```python
from build123d import *

# Parameters (mm, degrees)
SKETCH1_W           = 100
SKETCH1_H           = 75
BOSS_EXTRUDE1_DEPTH = 1.5875
SKETCH4_R           = 1.35
CUT_EXTRUDE1_DEPTH  = 2.5875


with BuildPart() as part:
    # Sketch1 → Boss-Extrude1 (new body)
    with BuildSketch(Plane(origin=(0, 0, 0), x_dir=(1, 0, 0), z_dir=(0, 1, 0))):
        with Locations((50, 37.5)):
            Rectangle(SKETCH1_W, SKETCH1_H)
    extrude(amount=BOSS_EXTRUDE1_DEPTH)

    # Sketch4 → Cut-Extrude1 (cut, through all)
    with BuildSketch(Plane(origin=(0, 1.5875, 0), x_dir=(1, 0, 0), z_dir=(0, 1, 0))):
        with Locations((10.86, 53.96)):
            Circle(SKETCH4_R)
        with Locations((10.86, 49.96)):
            Circle(SKETCH4_R)
        with Locations((10.86, 45.96)):
            Circle(SKETCH4_R)
        with Locations((14.86, 53.96)):
            Circle(SKETCH4_R)
        with Locations((14.86, 49.96)):
            Circle(SKETCH4_R)
        with Locations((14.86, 45.96)):
            Circle(SKETCH4_R)
        with Locations((18.86, 53.96)):
            Circle(SKETCH4_R)
        with Locations((18.86, 49.96)):
            Circle(SKETCH4_R)
        with Locations((18.86, 45.96)):
            Circle(SKETCH4_R)
        with Locations((34.86, 53.96)):
            Circle(SKETCH4_R)
        with Locations((34.86, 49.96)):
            Circle(SKETCH4_R)
        with Locations((34.86, 45.96)):
            Circle(SKETCH4_R)
        with Locations((38.86, 53.96)):
            Circle(SKETCH4_R)
        with Locations((38.86, 49.96)):
            Circle(SKETCH4_R)
        with Locations((38.86, 45.96)):
            Circle(SKETCH4_R)
        with Locations((42.86, 53.96)):
            Circle(SKETCH4_R)
        with Locations((42.86, 49.96)):
            Circle(SKETCH4_R)
        with Locations((42.86, 45.96)):
            Circle(SKETCH4_R)
        with Locations((58.86, 53.96)):
            Circle(SKETCH4_R)
        with Locations((58.86, 49.96)):
            Circle(SKETCH4_R)
        with Locations((58.86, 45.96)):
            Circle(SKETCH4_R)
        with Locations((62.86, 53.96)):
            Circle(SKETCH4_R)
        with Locations((62.86, 49.96)):
            Circle(SKETCH4_R)
        with Locations((62.86, 45.96)):
            Circle(SKETCH4_R)
        with Locations((66.86, 53.96)):
            Circle(SKETCH4_R)
        with Locations((66.86, 49.96)):
            Circle(SKETCH4_R)
        with Locations((66.86, 45.96)):
            Circle(SKETCH4_R)
        with Locations((82.86, 53.96)):
            Circle(SKETCH4_R)
        with Locations((82.86, 49.96)):
            Circle(SKETCH4_R)
        with Locations((82.86, 45.96)):
            Circle(SKETCH4_R)
        with Locations((86.86, 53.96)):
            Circle(SKETCH4_R)
        with Locations((86.86, 49.96)):
            Circle(SKETCH4_R)
        with Locations((86.86, 45.96)):
            Circle(SKETCH4_R)
        with Locations((90.86, 53.96)):
            Circle(SKETCH4_R)
        with Locations((90.86, 49.96)):
            Circle(SKETCH4_R)
        with Locations((90.86, 45.96)):
            Circle(SKETCH4_R)
    extrude(amount=-CUT_EXTRUDE1_DEPTH, mode=Mode.SUBTRACT)


solid = part.part
```
Design review of the part built by this model. Coordinates are the model's own, in mm. Coordinates: 2 decimals unless noted, no trailing zeros. Order: outer loops, then holes, each group sorted by start corner. A loop starts at its lowest first (then second) coordinate and runs counter-clockwise, first axis right, second up. Notation, with made-up numbers: (-29, 11) - (29, 11) arc R26 cw to (29, 42) - close; hole circle Ø8 at (-6, -14). An arc over 180 degrees is marked (long way). Answer in a Markdown table with one row per item.
(1) Wall thickness on line 1 along Z through (x, y) = (62.86, 0.9): over which ranges is the line inside the solid? List them lowest first. Write a range as from..to.
Checked values:
| item | result |
|---|---|
| line 1 | -75..-55.31, -52.61..-51.31, -48.61..-47.31, -44.61..0 |
(2) Consider section A-A on x = 34.86. State the section outline as (y, z) points, plus the area to 3 significant figures.
Checked values:
| item | result |
|---|---|
| outline | (0, -75) - (1.59, -75) - (1.59, -55.31) - (0, -55.31) - close; (0, -52.61) - (1.59, -52.61) - (1.59, -51.31) - (0, -51.31) - close; (0, -48.61) - (1.59, -48.61) - (1.59, -47.31) - (0, -47.31) - close; (0, -44.61) - (1.59, -44.61) - (1.59, 0) - (0, 0) - close |
| area | 106 mm^2 |
(3) Clearance check with a flat-ended pin moving along its axis: pin 1 (3 mm diameter, centred on x = 82.5, z = -28, fed in from -Y). State where the tip first meets the part, or that it passes through.
Checked values:
| item | result |
|---|---|
| pin 1 | y = 0 |
(4) Consider section B-B on y = 1.1. Give the number of separate pieces and of enclosed holes in the cut face, plus the area to 3 significant figures.
Checked values:
| item | result |
|---|---|
| separate pieces | 1 |
| enclosed holes | 36 |
| area | 7,290 mm^2 |
(5) The part is to be moulded in two halves that separate along X. For faces 1 (the cylindrical face through (85.51, 0.8, -54.02)), 2 (the flat face through (49, 0, -38)), say which applies: released by +X, released by -X, zero draft, split by the parting line, or undercut.
Checked values:
| item | result |
|---|---|
| face 1 | undercut |
| face 2 | zero draft |
